Geometry: see drawing. Coordinates: mm, zero at the bounding-box minimum. Round coordinates to 2 decimals unless told otherwise and drop trailing zeros. Write each loop counter-clockwise with the first axis right and the second up, starting at its lowest first coordinate (ties: lowest second). Pieces come first, ordered by that corner, then holes. Notation, with made-up numbers: (42.5, -7) -> (63.5, -7) arc R17 cw to (63.5, 9) -> close; hole circle Ø8 at (87, -9.75). An arc over 180 degrees is marked (long way). Write item = value, one per line.
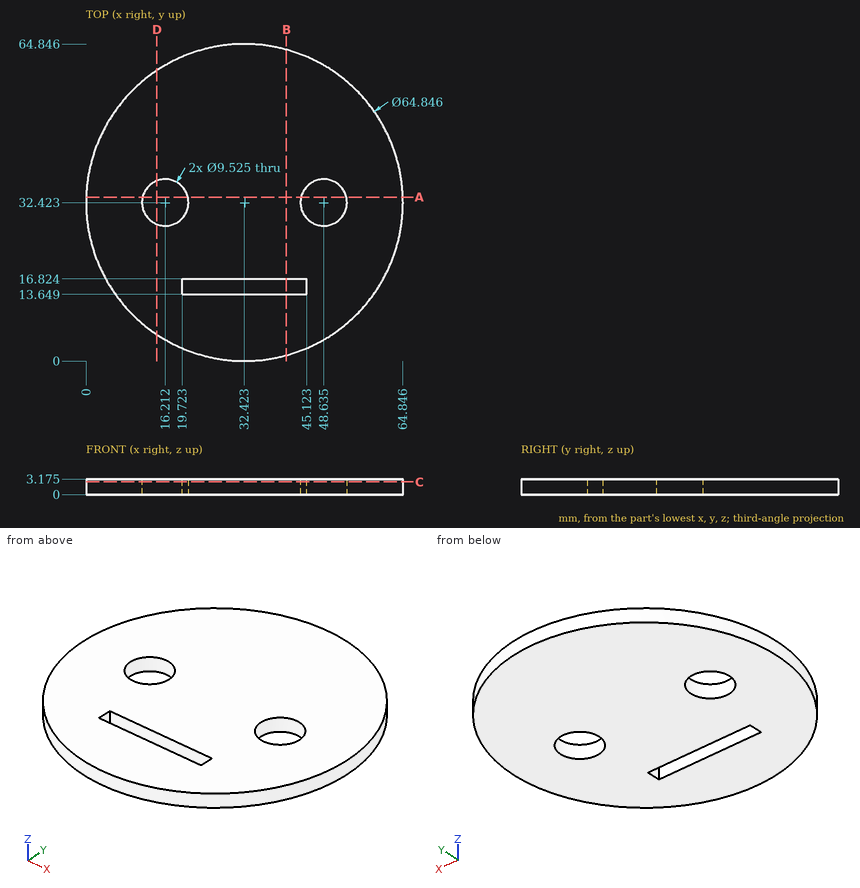
1) First-contact query: P1, Ø1.6, axis at y = 15.5, z = 1.5, coming from the +X side; P2, Ø1, axis at y = 15.5, z = 2, coming from the +X side; P3, Ø1, axis at x = 37, z = 0.5, coming from the -Y side. Flat tips, straight axial feed; report the tip coordinate or a pass-through.
Solutions:
P1 = 60.55
P2 = 60.38
P3 = 0.26
2) Cut plane D-D (x = 14.5). Return the cut outline in (y, z) (1 decimal).
Solutions:
outline = (5.4, 0) -> (28, 0) -> (28, 3.2) -> (5.4, 3.2) -> close; (36.9, 0) -> (59.4, 0) -> (59.4, 3.2) -> (36.9, 3.2) -> close
3) Cut plane B-B (x = 41). Return the cut outline in (y, z) (1 decimal).
Solutions:
outline = (1.2, 0) -> (13.6, 0) -> (13.6, 3.2) -> (1.2, 3.2) -> close; (16.8, 0) -> (63.7, 0) -> (63.7, 3.2) -> (16.8, 3.2) -> close
4) Line query: L1, parallel to Y at x = 33, z = 1.2 (1 decimal); L2, parallel to Y at x = 52.5, z = 1.8 (1 decimal); L3, parallel to X at y = 14.5, z = 2.85 (1 decimal). Output: solid intervals per line, ascending. Write a range as from..to.
Solutions:
L1 = 0..13.6, 16.8..64.8
L2 = 7..29.6, 35.2..57.9
L3 = 5.4..19.7, 45.1..59.4
5) Cut plane A-A (y = 33.5). Count the separate pieces of the cut face and the enclosed holes in it, and give its area (3 significant figures).
Solutions:
separate_pieces = 3
enclosed_holes = 0
area = 147 mm^2
6) Cut plane C-C (z = 2.6). Return the cut outline in (x, y) (1 decimal), and give its area (3 significant figures).
Solutions:
outline = circle Ø64.8 at (32.4, 32.4); hole circle Ø9.5 at (16.2, 32.4); hole (19.7, 13.6) -> (45.1, 13.6) -> (45.1, 16.8) -> (19.7, 16.8) -> close; hole circle Ø9.5 at (48.6, 32.4)
area = 3,080 mm^2
